Source: CAD feature listing. Evaluate the final solid. Frame: model axes, mm. A direction names the side the tool comes from. Round coordinates to 2 decimals unless told otherwise and drop trailing zeros. Loops run counter-clockwise (first coordinate to the right, second up) from the corner with the lowest first, then second, coordinate; pieces in that order, holes last.
Item 1: Section query C-C on x = 94.5. Return loops of the section in (y, z), then the cut area to 3 significant figures.
Item 2: Ray query, L1, parallel to X at y = 283, z = 39; L2, parallel to Y at x = 60, z = -1.4; L3, parallel to X at y = 40, z = 160.5. Return the intervals inside material, ascending.
Item 3: Section query B-B on y = 280. Return loops of the section in (x, z).
Item 4: Access query for faces 1 (the flat face through (275.06, 66.71, 88.71)), 2 (the flat face through (1.5, 287, 91)), 3 (the flat face through (-2, 148, 91)), 4 (the flat face through (300, 25, 89)). Directions: +Z, -Z, +X, -X, +Y, -Y. A direction counts if a zero-diameter tool reaches every point of the face in a straight line with its end or side. Return the directions, or none.
Item 5: Section query D-D on y = 41.5. Return loops of the section in (x, z).
Item 6: First-contact query: P1, Ø15, axis at y = 24.5, z = 113.5, coming from the -X side; P2, Ø1.5, axis at y = 379, z = 129, coming from the +X side; P3, Ø3, axis at y = 276.5, z = 99.5, coming from the +X side. Flat tips, straight axial feed; report the tip coordinate or a pass-through.
Item 7: Pull-direction query (Y, two-part tool) for faces 5 (the flat face through (56.602, 340.527, 91.26)), 6 (the flat face through (57.62, 339.84, 88.71)), 7 (the flat face through (92, 149, 182)); classes: released by +Y, released by -Y, zero draft, split by the parting line, or undercut.
```python
from build123d import *

# Parameters (mm, degrees)
EXTRUDE_3_DEPTH          = 180
EXTRUDE_4_DEPTH          = 2
EXTRUDE_5_DEPTH          = 180
CUT_EXTRUDE_8_DEPTH      = 6
CUT_EXTRUDE_8_DEPTH_BACK = 14
SKETCH_10_R              = 2.5
SKETCH_10_R_2            = 6
CUT_EXTRUDE_9_DEPTH      = 180
SKETCH_11_W              = 274.631033311
SKETCH_11_H              = 184
SKETCH_11_W_2            = 270.631033311
SKETCH_11_H_2            = 180
EXTRUDE_1_DEPTH          = 100
EXTRUDE_6_REACH          = 466.254
EXTRUDE_7_DEPTH          = 180
EXTRUDE_8_DEPTH          = 2
EXTRUDE_9_REACH          = 520.498
SKETCH_15_W              = 267.131033311
SKETCH_15_H              = 2


with BuildPart() as part:
    # Sketch 1 → Extrude 3 (new body)
    with BuildSketch(Plane.XY):
        with BuildLine():
            Line((300, 0), (0, 0))
            Line((0, 0), (0, 200))
            Line((0, 200), (270, 200))
            Line((270, 200), (241.796905997, 110.612978654))
            ThreePointArc((241.796905997, 110.612978654), (242.584644274, 109.746742593), (243.337981207, 108.850427931))
            Line((243.337981207, 108.850427931), (272.728222629, 202))
            Line((272.728222629, 202), (-2, 202))
            Line((-2, 202), (-2, -2))
            Line((-2, -2), (302, -2))
            Line((302, -2), (302, 51.154700538))
            Line((302, 51.154700538), (248.866473036, 81.831356634))
            ThreePointArc((248.866473036, 81.831356634), (248.571049064, 80.851494363), (248.242374569, 79.882278975))
            Line((248.242374569, 79.882278975), (300, 50))
            Line((300, 50), (300, 0))
        make_face()
    extrude(amount=EXTRUDE_3_DEPTH)

    # Sketch 7 → Extrude 4 (add)
    with BuildSketch(Plane(origin=(0, 0, 0), x_dir=(-1, 0, 0), z_dir=(0, 0, -1))):
        Polygon((-272.728222629, 202), (-275.433236518, 66.493028586), (-302, 51.154700538), (-302, -2), (2, -2), (2, 202), align=None)
    extrude_4 = extrude(amount=EXTRUDE_4_DEPTH)

    # Mirror 5: Extrude 4 across plane
    add(extrude_4.mirror(Plane.XY.offset(90)))

    # Sketch 8 → Extrude 5 (add)
    with BuildSketch(Plane.XY):
        with BuildLine():
            Line((191.022225211, 97.764571353), (0, 144.327661976))
            Line((0, 144.327661976), (0, 140.399780569))
            Line((0, 140.399780569), (190.270548779, 94.019916677))
            ThreePointArc((190.270548779, 94.019916677), (190.586734182, 95.904218314), (191.022225211, 97.764571353))
        make_face()
    extrude(amount=EXTRUDE_5_DEPTH)

    # Sketch 10 → Cut-Extrude 8 (cut, two sides: drawn at the far end of the back side and taken through both)
    with BuildSketch(Plane.XY.offset(-CUT_EXTRUDE_8_DEPTH_BACK)):
        with Locations(Location((60, 60, 0), (0, 0, 180))):
            Circle(SKETCH_10_R)
        with Locations(Location((95, 60, 0), (0, 0, 180))):
            Circle(SKETCH_10_R_2)
    extrude(amount=CUT_EXTRUDE_8_DEPTH + CUT_EXTRUDE_8_DEPTH_BACK, mode=Mode.SUBTRACT)

    # Sketch 8_3 → Cut-Extrude 9 (cut)
    with BuildSketch(Plane.XY):
        Polygon((0, 200), (270, 200), (270.631033311, 202), (0, 202), align=None)
    extrude(amount=CUT_EXTRUDE_9_DEPTH, mode=Mode.SUBTRACT)

    # Sketch 11 → Extrude 1 (add)
    with BuildSketch(Plane(origin=(0, 202, 0), x_dir=(1, 0, 0), z_dir=(0, 1, 0))):
        with Locations((135.315516656, -90)):
            Rectangle(SKETCH_11_W, SKETCH_11_H)
        with Locations((135.315516656, -90)):
            Rectangle(SKETCH_11_W_2, SKETCH_11_H_2, mode=Mode.SUBTRACT)
    extrude(amount=EXTRUDE_1_DEPTH)

    # Sketch 12 → Extrude 6 (add, up to next)
    with BuildSketch(Plane(origin=(0, 0, 180), x_dir=(-1, 0, 0), z_dir=(0, 0, -1)), mode=Mode.PRIVATE) as extrude_6_sk1:
        Polygon((-1.5, 302), (-1.5, 272), (-1, 262), (-3.5, 272), (-3.5, 302), align=None)
    extrude_6_tool1 = extrude(extrude_6_sk1.sketch, amount=EXTRUDE_6_REACH, mode=Mode.PRIVATE) - part.part
    add(extrude_6_tool1.solids().sort_by_distance((2.428571, 284.380952, 180))[0])

    # Sketch 13 → Extrude 7 (add)
    with BuildSketch(Plane(origin=(0, 0, 180), x_dir=(-1, 0, 0), z_dir=(0, 0, -1))):
        Polygon((-1.5, 302), (-113.268775045, 380.148175953), (-113.268775045, 378.749785823), (-3.5, 302), align=None)
        Polygon((111.768775045, 378.749785823), (111.768775045, 380.148175953), (0, 302), (2, 302), align=None)
    extrude(amount=EXTRUDE_7_DEPTH)

    # Sketch 14 → Extrude 8 (add)
    with BuildSketch(Plane(origin=(0, 0, 0), x_dir=(-1, 0, 0), z_dir=(0, 0, -1))):
        Polygon((-113.268775045, 380.148175953), (111.768775045, 380.148175953), (111.768775045, 378.749785823), (2, 302), (-3.5, 302), (-113.268775045, 378.749785823), align=None)
    extrude_8 = extrude(amount=EXTRUDE_8_DEPTH)

    # Mirror 6: Extrude 8 across plane
    add(extrude_8.mirror(Plane.XY.offset(90)))

    # Sketch 15 → Extrude 9 (add, up to next)
    with BuildSketch(Plane(origin=(0, 0, 180), x_dir=(-1, 0, 0), z_dir=(0, 0, -1)), mode=Mode.PRIVATE) as extrude_9_sk1:
        with Locations((-137.065516656, 301)):
            Rectangle(SKETCH_15_W, SKETCH_15_H)
    extrude_9_tool1 = extrude(extrude_9_sk1.sketch, amount=EXTRUDE_9_REACH, mode=Mode.PRIVATE) - part.part
    add(extrude_9_tool1.solids().sort_by_distance((137.065517, 301, 180))[0])


solid = part.part
```
Data:
1. outline: (-2, -2) - (54.02, -2) - (54.02, 0) - (0, 0) - (0, 180) - (117.36, 180) - (117.36, 0) - (65.98, 0) - (65.98, -2) - (302, -2) - (302, 182) - (-2, 182) - close; (365.63, -2) - (380.15, -2) - (380.15, 0) - (367.03, 0) - (367.03, 180) - (380.15, 180) - (380.15, 182) - (365.63, 182) - close; hole (121.29, 0) - (300, 0) - (300, 180) - (121.29, 180) - close
1. area: 2,930 mm2
2. L1: x = -2 to 0, 1.5 to 3.5, 270.63 to 272.63
2. L2: y = -2 to 57.5, 62.5 to 302, 341.5 to 380.15
2. L3: x = -2 to 0, 300 to 302
3. outline: (-2, -2) - (272.63, -2) - (272.63, 182) - (-2, 182) - close; hole (0, 0) - (1.5, 0) - (1.5, 180) - (0, 180) - close; hole (3.5, 0) - (270.63, 0) - (270.63, 180) - (3.5, 180) - close
4. face 1: +X
4. face 2: +Y
4. face 3: +Z, -Z, -X, -Y
4. face 4: none
5. outline: (-2, -2) - (302, -2) - (302, 182) - (-2, 182) - close; hole (0, 0) - (300, 0) - (300, 180) - (0, 180) - close
6. P1: stops at x = -2
6. P2: stops at x = 113.27
6. P3: stops at x = 272.63
7. face 5: released by +Y
7. face 6: undercut
7. face 7: zero draft
